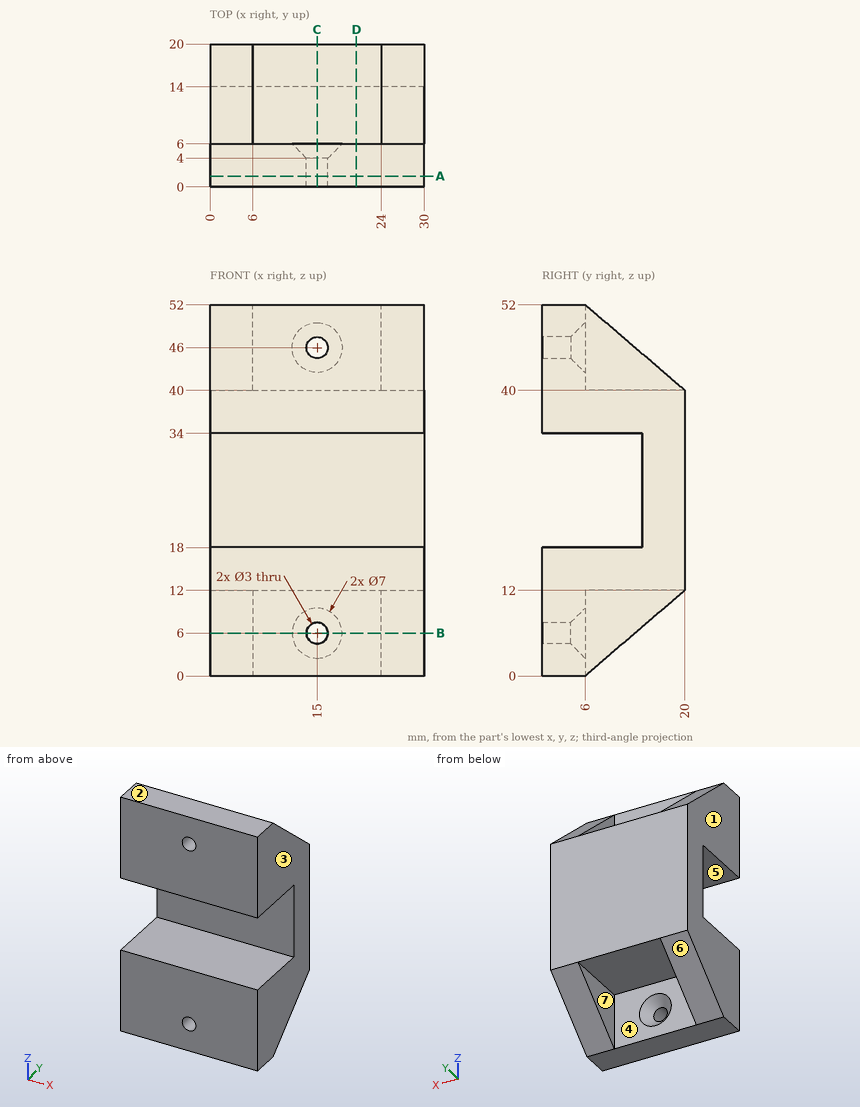
The drawing under review shows one solid part. Ordinate dimensions are in mm from its lowest x, y, z. A direction names the side the tool comes from. Give positions to 0.01 mm unless a question says otherwise; leave off trailing zeros. Order: outer loops, then holes, each group sorted by start corner. A loop starts at its lowest first (then second) coordinate and runs counter-clockwise, first axis right, second up. Notation, with made-up numbers: M 21.5,63.5 L 80.5,63.5 A18 cw 80.5,82.5 Z; hole C 88,0 d7. An arc over 180 degrees is marked long. Answer in a Markdown table with one row per item. Add a question column.
1. Add section C-C on x = 15. State the section outline as (y, z) points.
2. Add section D-D on x = 20.5. State the section outline as (y, z) points, plus the area to 3 significant figures.
3. Mouldability with a two-part tool opening along X and no side actions: class the marked faces 1, 2, 3 and 4 as released by +X, released by -X, zero draft, split by the parting line, or undercut.
4. Add section B-B on z = 6. State the section outline as (x, y) points.
5. For pin 1 Ø4 at (x, y) = (19.5, 14.5) entering from -Z; pin 2 Ø11 at (x, y) = (14.5, 15) entering from +Z; pin 3 Ø5 at (x, y) = (25, 15) entering from +Z; pin 4 Ø3.5 at (y, z) = (16, 47.5) entering from -X, all flat-tipped, find the tip position at first contact; note any pin that passes through.
6. Machinability: for the marked faces 5, 6 and 7, which of the approach directions +Z, -Z, +X, -X, +Y, -Y give a long, thin tool a straight path to every point of the face, cutting with its end or side? Answer none if there is none.
7. Add section A-A on y = 1.5. State the section outline as (x, z) points.
8. To check wall thickness, follow line 1 along X through (y, z) = (1.5, 46); line 2 along X through (y, z) = (18.5, 41); line 3 along Z through (x, y) = (12.5, 11.5). State the ranges of each line that lie inside material, in increasing order.
The answers:
| question | item | result |
|---|---|---|
| 1 | outline | M 0,0 L 6,0 L 6,2.5 L 4,4.5 L 0,4.5 Z; M 0,7.5 L 4,7.5 L 6,9.5 L 6,12 L 20,12 L 20,40 L 6,40 L 6,42.5 L 4,44.5 L 0,44.5 L 0,34 L 14,34 L 14,18 L 0,18 Z; M 0,47.5 L 4,47.5 L 6,49.5 L 6,52 L 0,52 Z |
| 2 | outline | M 0,0 L 6,0 L 6,12 L 20,12 L 20,40 L 6,40 L 6,52 L 0,52 L 0,34 L 14,34 L 14,18 L 0,18 Z |
| 2 | area | 480 mm2 |
| 3 | face 1 | released by -X |
| 3 | face 2 | zero draft |
| 3 | face 3 | released by +X |
| 3 | face 4 | undercut |
| 4 | outline | M 0,0 L 13.5,0 L 13.5,4 L 11.5,6 L 6,6 L 6,13 L 0,13 Z; M 16.5,0 L 30,0 L 30,13 L 24,13 L 24,6 L 18.5,6 L 16.5,4 Z |
| 5 | pin 1 | z = 12 |
| 5 | pin 2 | z = 40 |
| 5 | pin 3 | z = 46.43 |
| 5 | pin 4 | through |
| 6 | face 5 | +X, -X, -Y |
| 6 | face 6 | -Z, +X, -X, +Y |
| 6 | face 7 | -Z, +Y |
| 7 | outline | M 0,0 L 30,0 L 30,18 L 0,18 Z; M 0,34 L 30,34 L 30,52 L 0,52 Z; hole C 15,6 d3; hole C 15,46 d3 |
| 8 | line 1 | 0 to 13.5, 16.5 to 30 |
| 8 | line 2 | 0 to 6, 24 to 30 |
| 8 | line 3 | 12 to 18, 34 to 40 |
